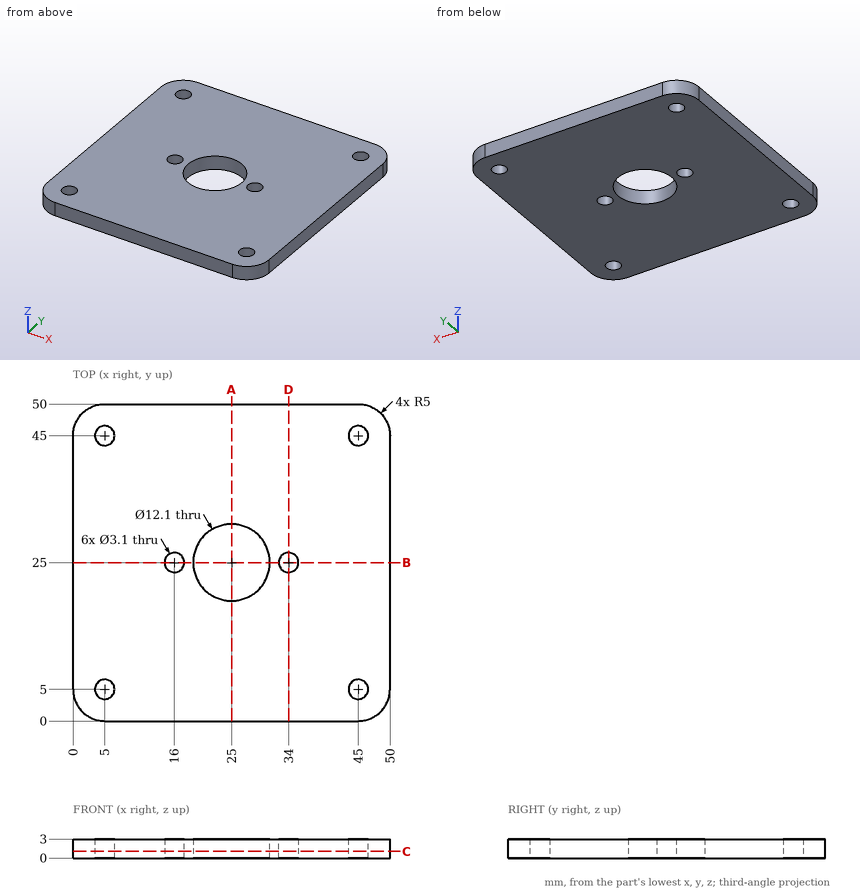
The figure shows three views and two pictorial views of one solid part (mm, origin at its lowest corner). Answer the questions. Give positions to 0.01 mm unless a question says otherwise; leave off trailing zeros. Write each loop counter-clockwise with the first axis right and the second up, starting at its lowest first coordinate (ties: lowest second). Pieces come first, ordered by that corner, then holes. Notation, with made-up numbers: (67, 43) - (124, 43) arc R31 ccw to (124, 74) - close; hole circle Ø2 at (-2.75, -38). An arc over 180 degrees is marked (long way). Use CSV: the item, a comma, the result in double quotes. Start each with the question number.
Item 1: The part is cut by section B-B, the plane y = 25. Give the vertices of the cut face in (x, z), and give its area (3 significant figures).
Item 2: Flat-ended cylindrical pins translate along their axes: P1, Ø5, axis at x = 45, y = 5, coming from the -Z side; P2, Ø2.5, axis at x = 5, y = 5, coming from the -Z side. Find the tip coordinate at first contact, or state that the pin passes through.
Item 3: The part is cut by section A-A, the plane x = 25. Give the vertices of the cut face in (y, z), and give its area (3 significant figures).
Item 4: The part is cut by section C-C, the plane z = 1.05. Give the vertices of the cut face in (x, y), and give its area (3 significant figures).
Item 5: Consider line 1 (Y direction, x = 5, z = 1.55); line 2 (Y direction, x = 4, z = 2.6); line 3 (Y direction, x = 34, z = 1.3). Determine where each line is inside the solid, lowest interval first.
Item 6: The part is cut by section D-D, the plane x = 34. Give the vertices of the cut face in (y, z).
Taken from the geometry:
1,outline,"(0, 0) - (14.45, 0) - (14.45, 3) - (0, 3) - close; (17.55, 0) - (18.95, 0) - (18.95, 3) - (17.55, 3) - close; (31.05, 0) - (32.45, 0) - (32.45, 3) - (31.05, 3) - close; (35.55, 0) - (50, 0) - (50, 3) - (35.55, 3) - close"
1,area,"95.1 mm2"
2,P1,"z = 0"
2,P2,"through"
3,outline,"(0, 0) - (18.95, 0) - (18.95, 3) - (0, 3) - close; (31.05, 0) - (50, 0) - (50, 3) - (31.05, 3) - close"
3,area,"114 mm2"
4,outline,"(0, 5) arc R5 ccw to (5, 0) - (45, 0) arc R5 ccw to (50, 5) - (50, 45) arc R5 ccw to (45, 50) - (5, 50) arc R5 ccw to (0, 45) - close; hole circle Ø3.1 at (5, 5); hole circle Ø3.1 at (5, 45); hole circle Ø3.1 at (16, 25); hole circle Ø12.1 at (25, 25); hole circle Ø3.1 at (34, 25); hole circle Ø3.1 at (45, 5); hole circle Ø3.1 at (45, 45)"
4,area,"2,320 mm2"
5,line 1,"0 to 3.45, 6.55 to 43.45, 46.55 to 50"
5,line 2,"0.1 to 3.82, 6.18 to 43.82, 46.18 to 49.9"
5,line 3,"0 to 23.45, 26.55 to 50"
6,outline,"(0, 0) - (23.45, 0) - (23.45, 3) - (0, 3) - close; (26.55, 0) - (50, 0) - (50, 3) - (26.55, 3) - close"
